```python
from build123d import *

# Parameters (mm, degrees)
SKETCH1_W            = 15
SKETCH1_H            = 6
BOSS_EXTRUDE1_DEPTH  = 2
BOSS_EXTRUDE2_DEPTH  = 2
BOSS_EXTRUDE3_DEPTH  = 2.25
SKETCH4_W            = 2
SKETCH4_H            = 6
CUT_EXTRUDE1_DEPTH   = 2.5
SKETCH7_W            = 4
SKETCH7_H            = 4.5
BOSS_EXTRUDE4_DEPTH  = 0.45
SKETCH14_W           = 0.5
SKETCH14_H           = 1.65
CUT_EXTRUDE5_DEPTH   = 2
SKETCH8_W            = 0.4
SKETCH8_H            = 3.371005291
BOSS_EXTRUDE5_DEPTH  = 0.75
CUT_EXTRUDE4_DEPTH   = 4.5
SKETCH12_W           = 1.6
SKETCH12_H           = 1.887701739
BOSS_EXTRUDE10_DEPTH = 0.75
FILLET1_R            = 2


with BuildPart() as part:
    # Sketch1 → Boss-Extrude1 (new body)
    with BuildSketch(Plane.XY):
        Rectangle(SKETCH1_W, SKETCH1_H)
    extrude(amount=BOSS_EXTRUDE1_DEPTH)

    # Sketch2 → Boss-Extrude2 (add)
    with BuildSketch(Plane.XY.offset(2)):
        with BuildLine():
            Line((-5.312816027, 1.330227393), (2.025172286, 1.330227393))
            ThreePointArc((2.025172286, 1.330227393), (3.334872121, 0.020527559), (2.025172286, -1.289172275))
            Line((2.025172286, -1.289172275), (-5.312816027, -1.289172275))
            ThreePointArc((-5.312816027, -1.289172275), (-6.622515861, 0.020527559), (-5.312816027, 1.330227393))
        make_face()
    extrude(amount=BOSS_EXTRUDE2_DEPTH)

    # Sketch3 → Boss-Extrude3 (add, symmetric)
    with BuildSketch(Plane(origin=(0, 0, 0), x_dir=(1, 0, 0), z_dir=(0, 1, 0))):
        with BuildLine():
            Line((-5.267009627, 0.659268098), (-4.040664768, 2.641993005))
            ThreePointArc((-4.040664768, 2.641993005), (-3.372127042, 4.157552016), (-3.143471892, 5.798155145))
            Line((-3.143471892, 5.798155145), (-3.143471892, 7.885245495))
            Line((-3.143471892, 7.885245495), (-3.143471892, 12.19944937))
            Line((-3.143471892, 12.19944937), (2.127297199, 12.19944937))
            Line((2.127297199, 12.19944937), (2.127297199, 7.885245495))
            Line((2.127297199, 7.885245495), (2.127297199, 4.714947067))
            Line((2.127297199, 4.714947067), (3.22873188, 1.042912685))
            Line((3.22873188, 1.042912685), (3.22873188, 0))
            Line((3.22873188, 0), (-5.267009627, 0))
            Line((-5.267009627, 0), (-5.267009627, 0.659268098))
        make_face()
    extrude(amount=BOSS_EXTRUDE3_DEPTH, both=True)

    # Sketch4 → Cut-Extrude1 (cut)
    with BuildSketch(Plane(origin=(7.5, 0, 0), x_dir=(0, 0, -1), z_dir=(1, 0, 0))):
        with Locations((-1, 0)):
            Rectangle(SKETCH4_W, SKETCH4_H)
    extrude(amount=-CUT_EXTRUDE1_DEPTH, mode=Mode.SUBTRACT)

    # Sketch7 → Boss-Extrude4 (add)
    with BuildSketch(Plane.ZY.offset(3.143471892)):
        with Locations((-10.19944937, 0)):
            Rectangle(SKETCH7_W, SKETCH7_H)
    extrude(amount=BOSS_EXTRUDE4_DEPTH)

    # Sketch14 → Cut-Extrude5 (cut)
    with BuildSketch(Plane(origin=(0, 0, 0), x_dir=(-1, 0, 0), z_dir=(0, 0, -1))):
        with Locations((5.017009627, 0)):
            Rectangle(SKETCH14_W, SKETCH14_H)
    extrude(amount=CUT_EXTRUDE5_DEPTH, mode=Mode.SUBTRACT)

    # Sketch8 → Boss-Extrude5 (add, symmetric)
    with BuildSketch(Plane(origin=(0, 0, 0), x_dir=(1, 0, 0), z_dir=(0, 1, 0))):
        with Locations((-7.3, 1.685502646)):
            Rectangle(SKETCH8_W, SKETCH8_H)
        with Locations((-5.3, 1.685502646)):
            Rectangle(SKETCH8_W, SKETCH8_H)
    extrude(amount=BOSS_EXTRUDE5_DEPTH, both=True)

    # Sketch11 → Cut-Extrude4 (cut)
    with BuildSketch(Plane(origin=(0, 2.25, 0), x_dir=(1, 0, 0), z_dir=(0, 1, 0))):
        with BuildLine():
            Line((-2.230616354, 12.19944937), (2.127297199, 12.19944937))
            Line((2.127297199, 12.19944937), (2.127297199, 7.412882239))
            ThreePointArc((2.127297199, 7.412882239), (-0.326306783, 9.556114202), (-2.230616354, 12.19944937))
        make_face()
    extrude(amount=-CUT_EXTRUDE4_DEPTH, mode=Mode.SUBTRACT)

    # Sketch12 → Boss-Extrude10 (add, symmetric)
    with BuildSketch(Plane(origin=(0, 0, 0), x_dir=(1, 0, 0), z_dir=(0, 1, 0))):
        with Locations((-6.3, 0.94385087)):
            Rectangle(SKETCH12_W, SKETCH12_H)
    extrude(amount=BOSS_EXTRUDE10_DEPTH, both=True)

    # Fillet1
    fillet1_edges = [part.edges().sort_by_distance(p)[0] for p in [
        (5, -3, 1),
        (5, 3, 1),
        (-7.5, -3, 1),
        (-7.5, 3, 1),
    ]]
    fillet(fillet1_edges, radius=FILLET1_R)


solid = part.part
```
Source: CAD feature listing. Evaluate the final solid. Frame: model axes, mm. A direction names the side the tool comes from. Round coordinates to 2 decimals unless told otherwise and drop trailing zeros. Write each loop counter-clockwise with the first axis right and the second up, starting at its lowest first coordinate (ties: lowest second). Pieces come first, ordered by that corner, then holes. Notation, with made-up numbers: M 71,18 L 107,18 A19 cw 107,46 Z; hole C 12,28 d9. An arc over 180 degrees is marked long. Answer as a JSON object with one key per item and string values. Group by question number.
(1) Section query B-B on x = -2.75. Output: boundary loops of the cut face in (y, z), then the cut area to 3 significant figures.
(2) Section query A-A on z = 1.5. Output: boundary loops of the cut face in (x, y).
(3) Mould query, pull axis X, two halves, no side actions, for faces 1 (the flat face through (-1, 2.25, -5)), 2 (the flat face through (-4.767, 0, -1)), 3 (the flat face through (2.127, 0, -6)), 4 (the cylindrical face through (-6.9, -2.43, 1.01)). Classes: +X half, -X half, draft (parallel to the pull), parting line (faces both ways), or undercut.
(4) Ray query, line 1 (X direction, y = -0.5, z = -2.25); line 2 (X direction, y = 0, z = 2.25); line 3 (Z direction, x = -3, y = -1.5). Return the intervals inside material, ascending. Write a range as [from, to].
(5) First-contact query: pin 1 (0.8 mm diameter, centred on y = 0.5, z = -6, fed in from +X); pin 2 (0.8 mm diameter, centred on x = -6.5, y = 0, fed in from -Z); pin 3 (1 mm diameter, centred on x = -2, z = 3.5, fed in from +Y). Flat tips, straight axial feed; report the tip coordinate or a pass-through.
(6) Reachability of faces 5 (the flat face through (-2, -1.289, 3)), 6 (the cylindrical face through (3.335, 0.049, 2.986)), 7 (the flat face through (-3.143, 0, -7)), 8 (the flat face through (-3.593, 0, -10)) from +Z, -Z, +X, -X, +Y, -Y: full face, straight path, thin tool, end or side. Return the list, or none.
(7) Section query C-C on y = 2. Output: boundary loops of the cut face in (x, z), then the cut area to 3 significant figures.
(8) Section query D-D on z = -6. Output: boundary loops of the cut face in (x, y).
Computed values:
{
 "1": {"outline": "M -3,0 L -2.25,0 L -2.25,-12.2 L 2.25,-12.2 L 2.25,0 L 3,0 L 3,2 L 1.33,2 L 1.33,4 L -1.29,4 L -1.29,2 L -3,2 Z", "area": "72.1 mm^2"},
 "2": {"outline": "M -7.5,-1 A2 ccw -5.5,-3 L 3,-3 A2 ccw 5,-1 L 5,1 A2 ccw 3,3 L -5.5,3 A2 ccw -7.5,1 Z"},
 "3": {"face 1": "draft", "face 2": "undercut", "face 3": "+X half", "face 4": "-X half"},
 "4": {"line 1": "[-7.5, -7.1], [-5.5, -5.1], [-4.28, 2.87]", "line 2": "[-6.62, 3.33]", "line 3": "[-12.2, 2]"},
 "5": {"pin 1": "x = 2.13", "pin 2": "z = -1.89", "pin 3": "y = 1.33"},
 "6": {"face 5": "+Z, +X, -X, -Y", "face 6": "+Z, +X", "face 7": "-X, +Y, -Y", "face 8": "-Z, -X, +Y, -Y"},
 "7": {"outline": "M -7.23,0 L -5.27,0 L -5.27,-0.66 L -4.04,-2.64 A6 cw -3.14,-5.8 L -3.14,-8.2 L -3.59,-8.2 L -3.59,-12.2 L -2.23,-12.2 A14.29 cw 2.13,-7.41 L 2.13,-4.71 L 3.23,-1.04 L 3.23,0 L 4.73,0 L 4.73,2 L -7.23,2 Z", "area": "86.5 mm^2"},
 "8": {"outline": "M -3.14,-2.25 L 2.13,-2.25 L 2.13,2.25 L -3.14,2.25 Z"}
}
